```python
from build123d import *

# Parameters (mm, degrees)
SKETCH1_R           = 26
BOSS_EXTRUDE1_DEPTH = 40
SKETCH2_R           = 3.5
CUT_EXTRUDE1_DEPTH  = 100


with BuildPart() as part:
    # Sketch1 → Boss-Extrude1 (new body)
    with BuildSketch(Plane.XY):
        with BuildLine():
            Line((40, 17), (45, 17))
            Line((45, 17), (45, 0))
            Line((45, 0), (-45, 0))
            Line((-45, 0), (-45, 17))
            Line((-45, 17), (-40, 17))
            Line((-40, 17), (-40, 45.637906937))
            Line((-40, 45.637906937), (-31.946191042, 45.637906937))
            ThreePointArc((-31.946191042, 45.637906937), (0, 68), (31.946191042, 45.637906937))
            Line((31.946191042, 45.637906937), (40, 45.637906937))
            Line((40, 45.637906937), (40, 17))
        make_face()
        with Locations((0, 34)):
            Circle(SKETCH1_R, mode=Mode.SUBTRACT)
    extrude(amount=BOSS_EXTRUDE1_DEPTH)

    # Sketch2 → Cut-Extrude1 (cut)
    with BuildSketch(Plane.XZ):
        with Locations((-35.5, 30.5)):
            Circle(SKETCH2_R)
        with Locations((-35.5, 9.5)):
            Circle(SKETCH2_R)
        with Locations((35.5, 30.5)):
            Circle(SKETCH2_R)
        with Locations((35.5, 9.5)):
            Circle(SKETCH2_R)
    extrude(amount=-CUT_EXTRUDE1_DEPTH, mode=Mode.SUBTRACT)


solid = part.part
```
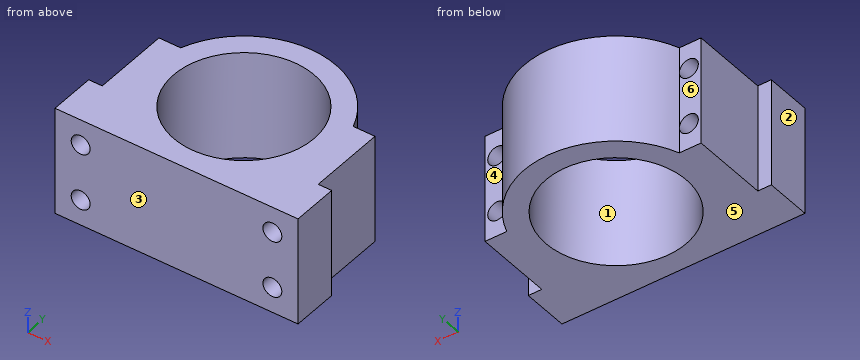
Could you check a few things on this model? Use its own coordinates, in mm. Face numbers are marked on the shaded views. A direction names the side the tool comes from. Coordinates: 2 decimals unless noted, no trailing zeros. Loops run counter-clockwise (first coordinate to the right, second up) from the corner with the lowest first, then second, coordinate; pieces in that order, holes last.
1) Will these pins go through, and if not, where does the flat tip stop? pin 1 Ø5.5 at (x, z) = (43, 14) entering from +Y; pin 2 Ø4 at (y, z) = (52, 19.5) entering from -X; pin 3 Ø6 at (x, z) = (34.5, 22.5) entering from +Y; pin 4 Ø6 at (x, y) = (2.5, 56.5) entering from -Z.
Reported:
pin 1: stops at y = 17
pin 2: stops at x = -30
pin 3: stops at y = 46.8
pin 4: passes through
2) Thinking about a two-plate mould opening in Y: for the marked faces 1, 2 and 3, which applies, released by +Y, released by -Y, zero draft, split by the parting line, or undercut?
Reported:
face 1: undercut
face 2: zero draft
face 3: released by -Y
3) Imagine slicing it at D-D (z = 35.5). List the corners of the cut face in (x, y) for me, and give its area (3 significant figures).
Reported:
outline: (-45, 0) - (45, 0) - (45, 17) - (40, 17) - (40, 45.64) - (31.95, 45.64) arc R34 ccw to (-31.95, 45.64) - (-40, 45.64) - (-40, 17) - (-45, 17) - close; hole circle Ø52 at (0, 34)
area: 2,740 mm2
4) Please list where these lines run through material, in increasing order: line 1 along X through (y, z) = (34.5, 15); line 2 along X through (y, z) = (22, 9); line 3 along Z through (x, y) = (35, 11).
Reported:
line 1: x = -40 to -26, 26 to 40
line 2: x = -40 to -38.96, -32.04 to -23.07, 23.07 to 32.04, 38.96 to 40
line 3: z = 0 to 6.04, 12.96 to 27.04, 33.96 to 40
5) Imagine slicing it at C-C (x = 0). List the corners of the cut face in (y, z) for me, and give its area (3 significant figures).
Reported:
outline: (0, 0) - (8, 0) - (8, 40) - (0, 40) - close; (60, 0) - (68, 0) - (68, 40) - (60, 40) - close
area: 640 mm2
6) Imagine slicing it at B-B (z = 9.5). List the corners of the cut face in (x, y) for me.
Reported:
outline: (-45, 0) - (-39, 0) - (-39, 45.64) - (-40, 45.64) - (-40, 17) - (-45, 17) - close; (-32, 0) - (32, 0) - (32, 45.64) - (31.95, 45.64) arc R34 ccw to (-31.95, 45.64) - (-32, 45.64) - close; (39, 0) - (45, 0) - (45, 17) - (40, 17) - (40, 45.64) - (39, 45.64) - close; hole circle Ø52 at (0, 34)
7) Imagine slicing it at A-A (y = 34). List the corners of the cut face in (x, z) for me, and give its area (3 significant figures).
Reported:
outline: (-40, 0) - (-26, 0) - (-26, 40) - (-40, 40) - close; (26, 0) - (40, 0) - (40, 40) - (26, 40) - close; hole circle Ø7 at (-35.5, 9.5); hole circle Ø7 at (-35.5, 30.5); hole circle Ø7 at (35.5, 9.5); hole circle Ø7 at (35.5, 30.5)
area: 966 mm2
8) Which directions (+Z, -Z, +X, -X, +Y, -Y) give clear straight access to the entire face, cutting with the end or side of a thin tool? Please do the marked faces 4, 5 and 6.
Reported:
face 4: +Z, -Z, +X, +Y
face 5: -Z, +X, -X, +Y, -Y
face 6: +Z, -Z, -X, +Y
